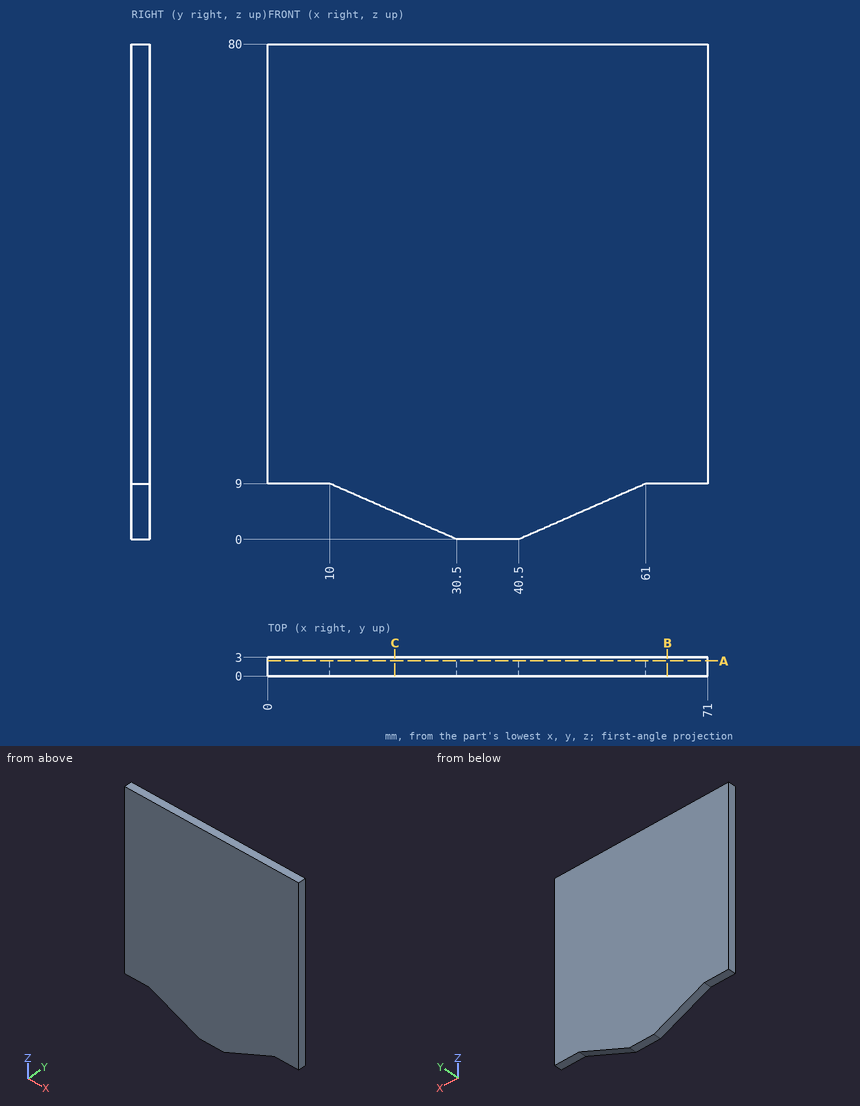
Part print with two shaded views. Sizes in mm from the minimum x, y, z corner. Round coordinates to 2 decimals unless told otherwise and drop trailing zeros. Loops run counter-clockwise (first coordinate to the right, second up) from the corner with the lowest first, then second, coordinate; pieces in that order, holes last.
1. Slice it at C-C (x = 20.5). Give the cut face in (y, z).
Solutions:
outline: (0, 4.39) - (3, 4.39) - (3, 80) - (0, 80) - close
2. Flat gauge pins, fed straight in: pin 1 (1.5 mm diameter, centred on x = 7, y = 2, fed in from -Z); pin 2 (1.5 mm diameter, centred on x = 24, y = 0.5, fed in from -Z). Where does each tip first touch, or does it go through?
Solutions:
pin 1: stops at z = 9
pin 2: stops at z = 2.52
3. Drill centre lines: line 1 along Z through (x, y) = (8.5, 2.35); line 2 along Z through (x, y) = (12.5, 2.65). Where is each one in solid material? Low to high.
Solutions:
line 1: z = 9 to 80
line 2: z = 7.9 to 80
4. Slice it at B-B (x = 64.5). Give the cut face in (y, z).
Solutions:
outline: (0, 9) - (3, 9) - (3, 80) - (0, 80) - close
5. Slice it at A-A (y = 2.45). Give the cut face in (x, z), and give its area (3 significant figures).
Solutions:
outline: (0, 9) - (10, 9) - (30.5, 0) - (40.5, 0) - (61, 9) - (71, 9) - (71, 80) - (0, 80) - close
area: 5,320 mm2
